Design review of the part built by this model. Coordinates are the model's own, in mm. Give positions to 0.01 mm unless a question says otherwise; leave off trailing zeros. Order: outer loops, then holes, each group sorted by start corner. A loop starts at its lowest first (then second) coordinate and runs counter-clockwise, first axis right, second up.
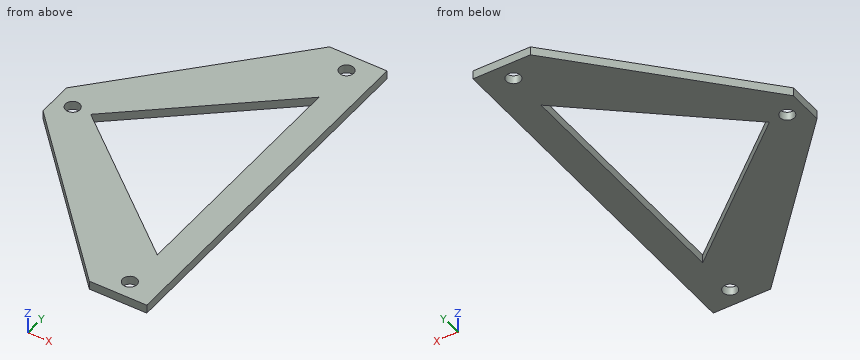
```python
from build123d import *

# Parameters (mm, degrees)
SKETCH1_W             = 8
SKETCH1_H             = 5
SKETCH1_R             = 1
BOSS_EXTRUDE1_DEPTH   = 1.2
SKETCH1_W_2           = 5
BOSS_EXTRUDE1_2_DEPTH = 1.2
BOSS_EXTRUDE1_3_DEPTH = 1.2
SKETCH2_W             = 5
SKETCH2_H             = 5
SKETCH2_R             = 1
BOSS_EXTRUDE4_DEPTH   = 1.2


with BuildPart() as part:
    # Sketch1 → Boss-Extrude1 (new body)
    with BuildSketch(Plane.XY):
        with Locations((35.73242964, 79.160231922)):
            Rectangle(SKETCH1_W, SKETCH1_H)
        with Locations((35.73242964, 79.160231922)):
            Circle(SKETCH1_R, mode=Mode.SUBTRACT)
    extrude(amount=BOSS_EXTRUDE1_DEPTH)



with BuildPart() as body_2:
    # Sketch1 → Boss-Extrude1 2 (new body)
    with BuildSketch(Plane.XY):
        with Locations((12.68242964, 102.210231922)):
            Rectangle(SKETCH1_W_2, SKETCH1_H)
        with Locations((12.68242964, 102.210231922)):
            Circle(SKETCH1_R, mode=Mode.SUBTRACT)
    extrude(amount=BOSS_EXTRUDE1_2_DEPTH)


with BuildPart() as body_3:
    # Sketch1 → Boss-Extrude1 3 (new body)
    with BuildSketch(Plane.XY):
        with Locations((35.73242964, 125.260231922)):
            Rectangle(SKETCH1_W, SKETCH1_H)
        with Locations((35.73242964, 125.260231922)):
            Circle(SKETCH1_R, mode=Mode.SUBTRACT)
    extrude(amount=BOSS_EXTRUDE1_3_DEPTH)


with BuildPart() as part_1:
    add(part.part)

    add(body_2.part)  # Boss-Extrude4 merges body 2

    add(body_3.part)  # Boss-Extrude4 merges body 3
    # Sketch2 → Boss-Extrude4 (add)
    # profile 1 of 6: a face of its own
    with BuildSketch(Plane.XY.offset(1.2)):
        Polygon((15.18242964, 99.710231922), (10.18242964, 99.710231922), (31.73242964, 76.660231922), (31.73242964, 81.660231922), (35.73242964, 81.660231922), (35.73242964, 85.008500761), (15.18242964, 102.210231922), align=None)
    # profile 2 of 6: a face of its own
    with BuildSketch(Plane.XY.offset(1.2)):
        Polygon((31.73242964, 127.760231922), (10.18242964, 104.710231922), (15.18242964, 104.710231922), (15.18242964, 102.210231922), (35.73242964, 119.411963083), (35.73242964, 122.760231922), (31.73242964, 122.760231922), align=None)
    # profile 3 of 6: a face of its own
    with BuildSketch(Plane.XY.offset(1.2)):
        with Locations((12.68242964, 102.210231922)):
            Rectangle(SKETCH2_W, SKETCH2_H)
        with Locations((12.68242964, 102.210231922)):
            Circle(SKETCH2_R, mode=Mode.SUBTRACT)
    # profile 4 of 6: a face of its own
    with BuildSketch(Plane.XY.offset(1.2)):
        Polygon((35.73242964, 119.411963083), (35.73242964, 85.008500761), (39.73242964, 81.660231922), (39.73242964, 122.760231922), align=None)
    # profile 5 of 6: a face of its own
    with BuildSketch(Plane.XY.offset(1.2)):
        Polygon((35.73242964, 122.760231922), (35.73242964, 119.411963083), (39.73242964, 122.760231922), align=None)
    # profile 6 of 6: a face of its own
    with BuildSketch(Plane.XY.offset(1.2)):
        Polygon((35.73242964, 85.008500761), (35.73242964, 81.660231922), (39.73242964, 81.660231922), align=None)
    extrude(amount=-BOSS_EXTRUDE4_DEPTH)


solid = part_1.part
```
1. Take a section at D-D (y = 81). State the section outline as (x, z) points.
Recorded:
outline: (27.68, 0) - (39.73, 0) - (39.73, 1.2) - (27.68, 1.2) - close
2. For line 1 along Y through (x, z) = (36.5, 0.8); line 2 along X through (y, z) = (102, 0.7); line 3 along Y through (x, z) = (36.25, 0.8), list the stretches that pass through material, from the lowest coordinate up.
Recorded:
line 1: y = 76.66 to 78.52, 79.8 to 124.62, 125.9 to 127.76
line 2: x = 10.18 to 11.7, 13.66 to 15.43, 35.73 to 39.73
line 3: y = 76.66 to 78.3, 80.02 to 124.4, 126.12 to 127.76
3. Take a section at B-B (y = 90). State the section outline as (x, z) points, then the cut area to 3 significant figures.
Recorded:
outline: (19.26, 0) - (29.77, 0) - (29.77, 1.2) - (19.26, 1.2) - close; (35.73, 0) - (39.73, 0) - (39.73, 1.2) - (35.73, 1.2) - close
area: 17.4 mm2
4. Take a section at A-A (x = 30). State the section outline as (y, z) points, then the cut area to 3 significant figures.
Recorded:
outline: (78.51, 0) - (89.81, 0) - (89.81, 1.2) - (78.51, 1.2) - close; (114.61, 0) - (125.91, 0) - (125.91, 1.2) - (114.61, 1.2) - close
area: 27.1 mm2
5. Take a section at C-C (z = 0.65). State the section outline as (x, y) points, then the cut area to 3 significant figures.
Recorded:
outline: (10.18, 99.71) - (31.73, 76.66) - (39.73, 76.66) - (39.73, 127.76) - (31.73, 127.76) - (10.18, 104.71) - close; hole circle Ø2 at (12.68, 102.21); hole (15.18, 102.21) - (35.73, 85.01) - (35.73, 119.41) - close; hole circle Ø2 at (35.73, 79.16); hole circle Ø2 at (35.73, 125.26)
area: 650 mm2
